Source: CAD feature listing. Evaluate the final solid. Frame: model axes, mm. A direction names the side the tool comes from. Round coordinates to 2 decimals unless told otherwise and drop trailing zeros. Loops run counter-clockwise (first coordinate to the right, second up) from the corner with the lowest first, then second, coordinate; pieces in that order, holes last.
Item 1: Ray query, L1, parallel to X at y = 2.35, z = -151; L2, parallel to Z at x = 89, y = 1.3; L3, parallel to X at y = 1.55, z = -111. Return the intervals inside material, ascending.
Item 2: First-contact query: P1, Ø1.5, axis at x = 87.5, y = 1, coming from the -Z side; P2, Ø0.9, axis at x = 51.5, y = 1, coming from the +Z side; P3, Ø0.9, axis at y = 2, z = -46, coming from the +X side; P4, Ø1.5, axis at x = 79.5, z = -104.5, coming from the -Y side. Flat tips, straight axial feed; report the tip coordinate or a pass-through.
Item 3: Section query D-D on z = -67. Return loops of the section in (x, y).
Item 4: Section query C-C on x = 30. Return loops of the section in (y, z).
Item 5: Section query A-A on z = -151. Return loops of the section in (x, y).
Item 6: Access query for faces 4 (the flat face through (90.5, 1, -8)), 5 (the flat face through (48, 1, -163.5)), 6 (the flat face through (40.5, 1, -1)), 7 (the flat face through (25.5, 1, -165)), 8 (the flat face through (15, 1, -2.5)). Directions: +Z, -Z, +X, -X, +Y, -Y. A direction counts if a zero-diameter tool reaches every point of the face in a straight line with its end or side. Return the directions, or none.
Item 7: Pull-direction query (X, two-part tool) for faces 1 (the flat face through (33, 1, -166.5)), 2 (the flat face through (55.5, 1, -1)), 3 (the flat face through (90.5, 1, -158)); classes: released by +X, released by -X, zero draft, split by the parting line, or undercut.
```python
from build123d import *

# Parameters (mm, degrees)
CROQUIS1_R              = 4.75
SALIENTE_EXTRUIR1_DEPTH = 3


with BuildPart() as part:
    # Croquis1 → Saliente-Extruir1 (new body)
    with BuildSketch(Plane(origin=(0, 0, 0), x_dir=(1, 0, 0), z_dir=(0, 1, 0))):
        Polygon((25.5, 2.5), (25.5, -0.5), (40.5, -0.5), (40.5, 2.5), (55.5, 2.5), (55.5, -0.5), (70.5, -0.5), (70.5, 2.5), (90.5, 2.5), (90.5, 13), (93.5, 13), (93.5, 33), (90.5, 33), (90.5, 53), (85.5, 53), (85.5, 113), (90.5, 113), (90.5, 133), (93.5, 133), (93.5, 153), (90.5, 153), (90.5, 163.5), (70.5, 163.5), (70.5, 166.5), (55.5, 166.5), (55.5, 163.5), (40.5, 163.5), (40.5, 166.5), (25.5, 166.5), (25.5, 163.5), (5.5, 163.5), (5.5, 153), (5.5, 133), (5.5, 113), (5.5, 93), (5.5, 73), (5.5, 53), (5.5, 33), (5.5, 13), (5.5, 2.5), align=None)
        with Locations(Location((30, 151, 0), (0, 0, 270))):
            Circle(CROQUIS1_R, mode=Mode.SUBTRACT)
    extrude(amount=SALIENTE_EXTRUIR1_DEPTH)


solid = part.part
```
Data:
1. L1: x = 5.5 to 25.25, 34.75 to 93.5
1. L2: z = -163.5 to -113, -53 to -2.5
1. L3: x = 5.5 to 85.5
2. P1: stops at z = -163.5
2. P2: stops at z = -2.5
2. P3: stops at x = 90.5
2. P4: stops at y = 0
3. outline: (5.5, 0) - (85.5, 0) - (85.5, 3) - (5.5, 3) - close
4. outline: (0, -166.5) - (3, -166.5) - (3, -155.75) - (0, -155.75) - close; (0, -146.25) - (3, -146.25) - (3, 0.5) - (0, 0.5) - close
5. outline: (5.5, 0) - (25.25, 0) - (25.25, 3) - (5.5, 3) - close; (34.75, 0) - (93.5, 0) - (93.5, 3) - (34.75, 3) - close
6. face 4: +Z, +X, +Y, -Y
6. face 5: -Z, +Y, -Y
6. face 6: +Z, +Y, -Y
6. face 7: -Z, -X, +Y, -Y
6. face 8: +Z, -X, +Y, -Y
7. face 1: zero draft
7. face 2: undercut
7. face 3: released by +X
